Verification items for the finished model (mm, model axes). A direction names the side the tool comes from. Round coordinates to 2 decimals unless told otherwise and drop trailing zeros. Write each loop counter-clockwise with the first axis right and the second up, starting at its lowest first coordinate (ties: lowest second). Pieces come first, ordered by that corner, then holes.
from build123d import *

# Parameters (mm, degrees)
F0_W     = 72.307944
F0_H     = 84.555768
F1_DEPTH = 74.3351
F2_R     = 15.279169
F3_DEPTH = 6.079547
F4_R     = 5.08
F5_W     = 29.425662
F5_H     = 21.301456
F6_DEPTH = 11.095189
F7_SIZE  = 5.08


with BuildPart() as f1:
    # F0 (on Top) → F1 (new body)
    with BuildSketch(Plane.XY):
        Rectangle(F0_W, F0_H)
    extrude(amount=F1_DEPTH)

    # F2 (on face) → F3 (join)
    with BuildSketch(Plane.XY.offset(74.3351)):
        with Locations((0, 16.862802)):
            Circle(F2_R)
    extrude(amount=F3_DEPTH)

    # F4
    f4_edges = [f1.edges().sort_by_distance(p)[0] for p in [
        (-15.279169, 16.862802, 80.414647),
        (0, -42.277884, 74.3351),
        (36.153972, 0, 74.3351),
        (36.153972, -42.277884, 37.16755),
    ]]
    fillet(f4_edges, radius=F4_R)

    # F5 (on face) → F6 (cut)
    with BuildSketch(Plane.YZ.offset(36.153972)):
        with Locations((-1.861071, 45.404758)):
            Rectangle(F5_W, F5_H)
    extrude(amount=-F6_DEPTH, mode=Mode.SUBTRACT)

    # F7
    f7_edges = [f1.edges().sort_by_distance(p)[0] for p in [
        (25.058783, -1.861071, 56.055486),
        (25.058783, -16.573902, 45.404758),
        (25.058783, -1.861071, 34.75403),
        (25.058783, 12.85176, 45.404758),
    ]]
    chamfer(f7_edges, length=F7_SIZE)


solid = f1.part
Q1. Tool access check on faces 1 (the flat face through (28.128, -14.563, 45.256)), 2 (the cylindrical face through (34.626, 3.096, 72.886)). Record the directions out of +Z, -Z, +X, -X, +Y, -Y that give a thin tool (end or side, any length) a straight path to the whole face; none if there is none.
Recorded:
face 1: +X
face 2: +Z, +X, +Y, -Y
Q2. Sectioned sample at D-D (y = -29). Enter the section's corners in (x, z).
Recorded:
outline: (-36.15, 0) - (36.15, 0) - (36.15, 69.26) arc R5.08 ccw to (31.07, 74.34) - (-36.15, 74.34) - close
Q3. Release check for a two-part mould opening along Z. For faces 3 (the flat face through (25.059, -2, 45)), 4 (the flat face through (-1, 1, 0)), 5 (the cylindrical face through (-11.26, 27.19, 74.83)), 6 (the flat face through (33, 12.852, 45)) record: released by +Z, released by -Z, zero draft, split by the parting line, or undercut.
Recorded:
face 3: undercut
face 4: released by -Z
face 5: zero draft
face 6: undercut
Q4. Sectioned sample at A-A (z = 44.5). Enter the section's corners in (x, y), plus the area to 3 significant figures.
Recorded:
outline: (-36.15, -42.28) - (31.07, -42.28) arc R5.08 ccw to (36.15, -37.2) - (36.15, -16.57) - (30.14, -16.57) - (25.06, -11.49) - (25.06, 7.77) - (30.14, 12.85) - (36.15, 12.85) - (36.15, 42.28) - (-36.15, 42.28) - close
area: 5,810 mm2
Q5. Material ranges on line 1 along Z through (x, y) = (6.5, 2); line 2 along X through (y, z) = (-2.5, 71); line 3 along X through (y, z) = (8.5, 53.5), recorded low to high.
Recorded:
line 1: z = 0 to 74.34
line 2: x = -36.15 to 35.84
line 3: x = -36.15 to 27.58
Q6. Sectioned sample at C-C (x = 26.5). Enter the section's corners in (y, z), plus the area to 3 significant figures.
Recorded:
outline: (-42.28, 0) - (42.28, 0) - (42.28, 74.34) - (-37.2, 74.34) arc R5.08 ccw to (-42.28, 69.26) - close; hole (-12.94, 38.39) - (9.21, 38.39) - (9.21, 52.42) - (-12.94, 52.42) - close
area: 5,970 mm2
Q7. Depth check by flat-ended pin: P1, Ø12, axis at y = 8, z = 35.5, coming from the +X side; P2, Ø3.5, axis at y = -5, z = 46.5, coming from the +X side; P3, Ø6.5, axis at x = 34, y = -3.5, coming from the +Z side. Enter the tip coordinate at first touch or a pass-through.
Recorded:
P1: stops at x = 36.15
P2: stops at x = 25.06
P3: stops at z = 74.34
Q8. Sectioned sample at B-B (y = -5). Enter the section's corners in (x, z).
Recorded:
outline: (-36.15, 0) - (36.15, 0) - (36.15, 34.75) - (30.14, 34.75) - (25.06, 39.83) - (25.06, 50.98) - (30.14, 56.06) - (36.15, 56.06) - (36.15, 69.26) arc R5.08 ccw to (31.07, 74.34) - (-36.15, 74.34) - close
